Input: part model. Units: mm. Frame: model coordinates. A direction names the side the tool comes from. Round coordinates to 2 decimals unless told otherwise and drop trailing zeros. Order: outer loops, then holes, each group sorted by start corner. A loop starts at its lowest first (then second) coordinate and runs counter-clockwise, first axis right, second up. Notation, with made-up numbers: (-6, 54) - (9, 54) arc R14 ccw to (9, 77) - close; hole circle Ø2 at (18, 48). An arc over 180 degrees is marked (long way). One line per item, written item: value. Start each with the question number.
from build123d import *

# Parameters (mm, degrees)
F1_DEPTH = 19.812
F2_R     = 5
F3_DEPTH = 29.972


with BuildPart() as f1:
    # F0 (on Front) → F1 (new body)
    with BuildSketch(Plane.XZ):
        with BuildLine():
            add(Edge.make_bspline(
                [(-57.2814941406, -25.2774953842), (-55.4948378039, -2.6600567826), (-53.3099503119, 24.9986247928), (-48.7638040936, 24.0367135251), (-47.9351952672, 23.8613896072)],
                knots=[0, 0, 0, 0, 0.8177337933, 1, 1, 1, 1], degree=3))
            Line((-57.2814941406, -25.2774953842), (0, -25.2774953842))
            add(Edge.make_bspline(
                [(-10.691601783, 23.8613896072), (-9.820200524, 24.2031852968), (-5.0967860131, 26.0558825509), (-2.289435327, -2.2189544531), (0, -25.2774953842)],
                knots=[0, 0, 0, 0, 0.1844854516, 1, 1, 1, 1], degree=3))
            Line((-10.691601783, 23.8613896072), (-47.9351952672, 23.8613896072))
        make_face()
    extrude(amount=F1_DEPTH)

    # F2 (on Top) → F3 (cut)
    with BuildSketch(Plane.XY):
        with Locations((-30.0922561437, -9.8419375718)):
            Circle(F2_R)
    extrude(amount=F3_DEPTH, mode=Mode.SUBTRACT)


solid = f1.part
1. Section A-A (x = -28). Return the cut outline in (y, z), then the cut area to 3 significant figures.
2. Pin query (flat end, axial travel): pin 1 (8 mm diameter, centred on x = -17, y = -8, fed in from +Z); pin 2 (3 mm diameter, centred on x = -29, y = -8, fed in from +Z); pin 3 (1 mm diameter, centred on y = -4.5, z = 17.5, fed in from +X). Return the tip coordinate at first contact, or that it passes through.
3. Set-up query: faces 3 (the face through (-28, 0, 1)), 4 (the face through (-34.06, -12.884, 11.764)), 5 (the face through (-24.9, -9.8, 23.861)). Return all of +Z, -Z, +X, -X, +Y, -Y with unobstructed straight access to the full face (end or side cutting, diameter ignored); none if empty.
4. Pull-direction query (X, two-part tool) for faces 1 (the face through (-30, -10, 0)), 2 (the face through (-28, -19.812, 1)); classes: released by +X, released by -X, zero draft, split by the parting line, or undercut.
5. Line query: line 1 (Z direction, x = -41, y = -10); line 2 (Z direction, x = -31, y = -5.75); line 3 (X direction, y = -9.75, z = 14). Output: solid intervals per line, ascending. Write a range as from..to.
Solved:
1. outline: (-19.81, -25.28) - (0, -25.28) - (0, 23.86) - (-5.3, 23.86) - (-5.3, 0) - (-14.38, 0) - (-14.38, 23.86) - (-19.81, 23.86) - close
1. area: 757 mm²
2. pin 1: stops at z = 23.86
2. pin 2: stops at z = 0
2. pin 3: stops at x = -5.41
3. face 3: +Z, -Z, +X, -X, +Y
3. face 4: +Z
3. face 5: +Z, +Y, -Y
4. face 1: undercut
4. face 2: zero draft
5. line 1: z = -25.28..23.86
5. line 2: z = -25.28..0
5. line 3: x = -53.29..-35.09, -25.09..-4.78
